```python
from build123d import *

# Parameters (mm, degrees)
F1_DEPTH = 90
F2_R     = 5
F3_DEPTH = 50
F4_W     = 30
F4_H     = 134.1311782598
F5_DEPTH = 40
F7_W     = 309.0550526977
F7_H     = 293.745405972
F8_DEPTH = 60
F9_SIZE  = 12


# Not quite as in the source:
# - a pattern or mirror of a feature is missing from the dataset's text; its kind, count and spacing are read off the source's solid


with BuildPart() as f1:
    # F0 (on Front) → F1 (new body, symmetric)
    with BuildSketch(Plane.XZ):
        Polygon((0, 65.2183964849), (0, 205), (-35, 205), (-35, 30), (-60, 30), (-60, 0), (0, 0), (60, 0), (60, 30), (35, 30), (35, 65.2183964849), align=None)
    extrude(amount=F1_DEPTH, both=True)

    # F2 (on Right) → F3 (cut, symmetric)
    with BuildSketch(Plane.YZ):
        with Locations((0, 155)):
            Circle(F2_R)
    extrude(amount=F3_DEPTH, both=True, mode=Mode.SUBTRACT)

    # F4 (on face) → F5 (cut, symmetric)
    with BuildSketch(Plane.XY.offset(30)):
        with Locations((20, 0)):
            Rectangle(F4_W, F4_H)
    extrude(amount=F5_DEPTH, both=True, mode=Mode.SUBTRACT)

    # F7 (on face) → F8 (cut)
    with BuildSketch(Plane(origin=(0, 87.2861679354, 15.3909064497), x_dir=(-1, 0, 0), z_dir=(0, 0.984807753, 0.1736481777))):
        with Locations((10.5363130569, 83.1948332489)):
            Rectangle(F7_W, F7_H)
    f8 = extrude(amount=F8_DEPTH, mode=Mode.SUBTRACT)

    # F8_copies: F8 across plane
    add(f8.mirror(Plane(origin=(0, 0, 0), x_dir=(0, 0, -1), z_dir=(0, -1, 0))), mode=Mode.SUBTRACT)

    # F9
    f9_edges = [f1.edges().sort_by_distance(p)[0] for p in [
        (0, 66.176603, 135.109198),
        (-35, 69.28158, 117.5),
        (-60, 87.355095, 15),
        (60, 87.355095, 15),
        (-60, 0, 30),
        (60, 0, 30),
        (0, -66.176603, 135.109198),
        (60, -87.355095, 15),
        (-35, -69.28158, 117.5),
        (-60, -87.355095, 15),
    ]]
    chamfer(f9_edges, length=F9_SIZE)


solid = f1.part
```
Here's how the part is built. I have some questions about the finished solid (model axes, mm). A direction names the side the tool comes from. Round coordinates to 2 decimals unless told otherwise and drop trailing zeros. Order: outer loops, then holes, each group sorted by start corner. A loop starts at its lowest first (then second) coordinate and runs counter-clockwise, first axis right, second up. Notation, with made-up numbers: (86, 61) -> (93, 61) arc R23 cw to (93, 76) -> close; hole circle Ø9 at (-34.75, -32.5). An arc over 180 degrees is marked (long way). Use a Markdown table: item, result. Add a question column.
(1) Suppose I cut it at A-A, the plane y = 10. Please give me the cut outline in (x, z).
(2) For pin 1 Ø8 at (x, z) = (31, 64) entering from -Y; pin 2 Ø19.5 at (y, z) = (-72, 41) entering from +X; pin 3 Ø1.5 at (y, z) = (-5, 76) entering from +X; pin 4 Ø6 at (y, z) = (0, 155) entering from -X, each with a flat end and sliding along its axis, tell me the tip position at first contact or that it passes through.
(3) Suppose I cut it at B-B, the plane x = 15. Please give me the cut outline in (y, z), and give its area (3 significant figures).
(4) Suppose I cut it at D-D, the plane x = -26. Please give me the cut outline in (y, z).
(5) I need wall thicknesses on line 1 along Z through (x, y) = (-23, 0); line 2 along X through (y, z) = (-42, 30.5); line 3 along X through (y, z) = (45, 9.5). Which ranges of each line are inside material? Lowest first, please.
(6) For faces 5 (the face through (35, 74, 47)), 6 (the face through (-35, -1, 99)), 7 (the face through (20, 67.066, 33)), which set-ups out of +Z, -Z, +X, -X, +Y, -Y let a thin tool reach every point of the face, with its end or its side?
(7) Suppose I cut it at C-C, the plane z = 155. Please give me the cut outline in (x, y), and give its area (3 significant figures).
(8) If we mould it in two halves opening along X, with no side actions, what happens to faces 1 (the face through (20, -67.066, 33)), 2 (the face through (42, -1, 30)), 3 (the face through (54.084, 81.401, 13.734)), 4 (the face through (-54.1, 81.9, 10.8))? For each: released by +X, released by -X, zero draft, split by the parting line, or undercut.
Verdict:
| question | item | result |
|---|---|---|
| 1 | outline | (-60, 0) -> (5, 0) -> (5, 65.22) -> (0, 65.22) -> (0, 205) -> (-35, 205) -> (-35, 30) -> (-48, 30) -> (-60, 18) -> close; (35, 0) -> (60, 0) -> (60, 18) -> (48, 30) -> (35, 30) -> close |
| 2 | pin 1 | y = -79.42 |
| 2 | pin 2 | x = 35 |
| 2 | pin 3 | x = 0 |
| 2 | pin 4 | through |
| 3 | outline | (-90, 0) -> (-67.07, 0) -> (-67.07, 65.22) -> (-78.5, 65.22) -> close; (67.07, 0) -> (90, 0) -> (78.5, 65.22) -> (67.07, 65.22) -> close |
| 3 | area | 2,240 mm2 |
| 4 | outline | (-90, 0) -> (90, 0) -> (84.71, 30) -> (81.66, 30) -> (50.81, 205) -> (-50.81, 205) -> (-81.66, 30) -> (-84.71, 30) -> close; hole circle Ø10 at (0, 155) |
| 5 | line 1 | 0 to 150, 160 to 205 |
| 5 | line 2 | -35 to 5 |
| 5 | line 3 | -60 to 5, 35 to 60 |
| 6 | face 5 | +Z, +X, +Y, -Y |
| 6 | face 6 | +Z, -X, +Y, -Y |
| 6 | face 7 | +Z, -Z |
| 7 | outline | (-35, -50.48) -> (-23, -62.67) -> (-12, -62.67) -> (0, -50.48) -> (0, -5) -> (-35, -5) -> close; (-35, 5) -> (0, 5) -> (0, 50.48) -> (-12, 62.67) -> (-23, 62.67) -> (-35, 50.48) -> close |
| 7 | area | 3,740 mm2 |
| 8 | face 1 | undercut |
| 8 | face 2 | zero draft |
| 8 | face 3 | released by +X |
| 8 | face 4 | released by -X |
